Design review of the part built by this model. Coordinates are the model's own, in mm. Give positions to 0.01 mm unless a question says otherwise; leave off trailing zeros. Loops run counter-clockwise (first coordinate to the right, second up) from the corner with the lowest first, then second, coordinate; pieces in that order, holes last. Notation, with made-up numbers: (62.5, 81) -> (91.5, 81) arc R30 ccw to (91.5, 118) -> close; hole circle Ø2 at (42, -32). An arc over 180 degrees is marked (long way). Answer in a Markdown table with one row per item. Add a question column.
(1) For pin 1 (12 mm diameter, centred on x = -1, z = 13, fed in from -Y); pin 2 (12 mm diameter, centred on y = 365.5, z = -19, fed in from -X); pin 3 (1.5 mm diameter, centred on y = 346.5, z = 6.5, fed in from -X); pin 4 (8 mm diameter, centred on x = -7.5, z = -8.5, fed in from -Y), all flat-tipped, find the tip position at first contact; note any pin that passes through.
(2) For line 1 (Y direction, x = 4.5, z = 14); line 2 (Y direction, x = 4.5, z = 7.5); line 3 (Y direction, x = -7, z = 10), list the stretches that pass through material, from the lowest coordinate up.
(3) Consider section A-A on x = -5. Write out the cut boundary in (y, z) (3 decimals).
(4) Consider section B-B on y = -15. Write out the cut boundary in (x, z), then the cut area to 3 significant figures.
from build123d import *

# Parameters (mm, degrees)
F0_R          = 25.4
F0_R_2        = 15.875
F2_DEPTH      = 12.7
F3_DEPTH      = 12.7
F1_R          = 12.7
F4_DEPTH      = 42.6116161379
F4_DEPTH_BACK = 575.7942935499


with BuildPart() as f2:
    # F0 (on Right) → F2 (new body, symmetric)
    with BuildSketch(Plane.YZ):
        with Locations((-63.608661294, 0)):
            Circle(F0_R)
        with Locations((-63.608661294, 0)):
            Circle(F0_R_2, mode=Mode.SUBTRACT)
    extrude(amount=F2_DEPTH, both=True)



with BuildPart() as f3:
    # F0 (on Right) → F3 (new body, symmetric)
    with BuildSketch(Plane.YZ):
        with Locations((596.791338706, 0)):
            Circle(F0_R)
        with Locations((596.791338706, 0)):
            Circle(F0_R_2, mode=Mode.SUBTRACT)
    extrude(amount=F3_DEPTH, both=True)


with BuildPart() as f2_1:
    add(f2.part)

    add(f3.part)  # F4 merges F3
    # F1 (on Front) → F4 (join, two sides)
    with BuildSketch(Plane.XZ) as f4_sk:
        Circle(F1_R)
    extrude(amount=F4_DEPTH)
    extrude(f4_sk.sketch, amount=-F4_DEPTH_BACK)


solid = f2_1.part
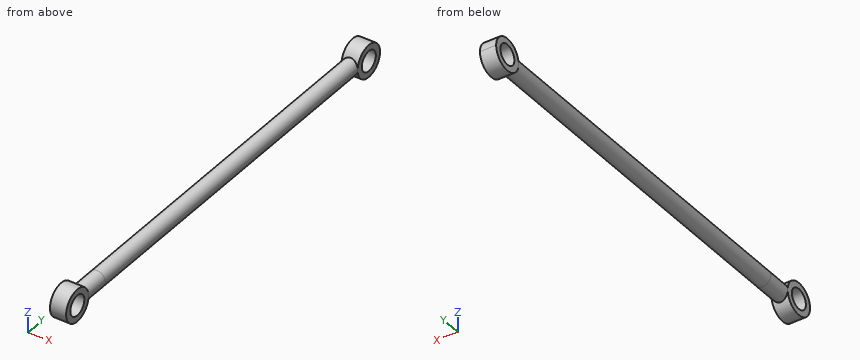
Values follow:
| question | item | result |
|---|---|---|
| 1 | pin 1 | y = -88.03 |
| 1 | pin 2 | through |
| 1 | pin 3 | x = -11.32 |
| 1 | pin 4 | y = -88.61 |
| 2 | line 1 | -84.8 to -71.09, -56.12 to -42.42, 575.6 to 589.31, 604.28 to 617.98 |
| 2 | line 2 | -87.88 to -77.6, -49.62 to 582.8, 610.78 to 621.06 |
| 2 | line 3 | -86.96 to -75.94, -51.28 to 584.46, 609.12 to 620.14 |
| 3 | outline | (-41.051, -11.674) -> (574.233, -11.674) arc R25.4 ccw (long way) to (574.233, 11.674) -> (-41.051, 11.674) arc R25.4 ccw (long way) to start; hole circle Ø31.75 at (-63.609, 0); hole circle Ø31.75 at (596.791, 0) |
| 4 | outline | circle Ø25.4 at (0, 0) |
| 4 | area | 507 mm2 |
